from build123d import *

# Parameters (mm, degrees)
SKETCH_1_W               = 420
SKETCH_1_H               = 420
EXTRUDE_1_DEPTH          = 5
SKETCH_3_W               = 50
SKETCH_3_H               = 10
SKETCH_3_W_2             = 10
SKETCH_3_H_2             = 50
EXTRUDE_2_DEPTH          = 10
SKETCH_4_W               = 200
SKETCH_4_H               = 10
SKETCH_4_W_2             = 10
SKETCH_4_H_2             = 200
EXTRUDE_3_DEPTH          = 10
FILLET_1_R               = 5
SKETCH_5_R               = 2
CUT_EXTRUDE_1_DEPTH      = 422.366823564
SKETCH_6_R               = 2
CUT_EXTRUDE_2_DEPTH      = 375.733238451
CUT_EXTRUDE_3_DEPTH      = 422.366823564
CUT_EXTRUDE_3_DEPTH_BACK = 422.366823564
SKETCH_7_R               = 2
SKETCH_8_R               = 2
CUT_EXTRUDE_4_DEPTH      = 375.733238451
CUT_EXTRUDE_5_DEPTH      = 422.366823564
CUT_EXTRUDE_5_DEPTH_BACK = 422.366823564
SKETCH_9_R               = 2
SKETCH_10_R              = 2
CUT_EXTRUDE_6_DEPTH      = 375.733238451
CUT_EXTRUDE_7_DEPTH      = 422.366823564
CUT_EXTRUDE_7_DEPTH_BACK = 422.366823564
SKETCH_11_R              = 2
SKETCH_12_R              = 2
CUT_EXTRUDE_8_DEPTH      = 375.733238451
SCALE_1_SCALE            = 0.5


with BuildPart() as part:
    # 草图1 → 凸台-拉伸1 (new body)
    with BuildSketch(Plane.XY):
        Rectangle(SKETCH_1_W, SKETCH_1_H)
    extrude(amount=EXTRUDE_1_DEPTH)

    # 草图3 → 凸台-拉伸2 (add)
    with BuildSketch(Plane(origin=(0, 0, 0), x_dir=(-1, 0, 0), z_dir=(0, 0, -1))):
        with Locations((-130, -205)):
            Rectangle(SKETCH_3_W, SKETCH_3_H)
        with Locations((-205, -130)):
            Rectangle(SKETCH_3_W_2, SKETCH_3_H_2)
        with Locations((-205, 130)):
            Rectangle(SKETCH_3_W_2, SKETCH_3_H_2)
        with Locations((-130, 205)):
            Rectangle(SKETCH_3_W, SKETCH_3_H)
        with Locations((205, 130)):
            Rectangle(SKETCH_3_W_2, SKETCH_3_H_2)
        with Locations((130, 205)):
            Rectangle(SKETCH_3_W, SKETCH_3_H)
        with Locations((205, -130)):
            Rectangle(SKETCH_3_W_2, SKETCH_3_H_2)
        with Locations((130, -205)):
            Rectangle(SKETCH_3_W, SKETCH_3_H)
    extrude(amount=EXTRUDE_2_DEPTH)

    # 草图4 → 凸台-拉伸3 (add)
    with BuildSketch(Plane.XY.offset(5)):
        with Locations((0, -205)):
            Rectangle(SKETCH_4_W, SKETCH_4_H)
        with Locations((205, 0)):
            Rectangle(SKETCH_4_W_2, SKETCH_4_H_2)
        with Locations((0, 205)):
            Rectangle(SKETCH_4_W, SKETCH_4_H)
        with Locations((-205, 0)):
            Rectangle(SKETCH_4_W_2, SKETCH_4_H_2)
    extrude(amount=EXTRUDE_3_DEPTH)

    # 圆角1
    fillet_1_edges = [part.edges().sort_by_distance(p)[0] for p in [
        (-210, 0, 15),
        (-200, 0, 15),
        (0, -210, 15),
        (0, -200, 15),
        (0, 200, 15),
        (0, 210, 15),
        (200, 0, 15),
        (210, 0, 15),
        (200, -130, -10),
        (210, -130, -10),
        (130, 210, -10),
        (130, 200, -10),
        (200, 130, -10),
        (210, 130, -10),
        (-130, -210, -10),
        (-130, -200, -10),
        (-130, 210, -10),
        (-130, 200, -10),
        (-210, 130, -10),
        (-200, 130, -10),
        (-210, -130, -10),
        (-200, -130, -10),
        (130, -210, -10),
        (130, -200, -10),
    ]]
    fillet(fillet_1_edges, radius=FILLET_1_R - 0.0001)  # a hair under: the kernel refuses the full size

    # 草图5 → 切除-拉伸1 (cut, through all)
    with BuildSketch(Plane(origin=(0, 155, 0), x_dir=(1, 0, 0), z_dir=(0, 1, 0))):
        with Locations(Location((205, 5, 0), (0, 0, 270))):
            Circle(SKETCH_5_R)
    extrude(amount=-CUT_EXTRUDE_1_DEPTH, mode=Mode.SUBTRACT)

    # 草图6 → 切除-拉伸2 (cut, through all)
    with BuildSketch(Plane(origin=(0, 100, 0), x_dir=(1, 0, 0), z_dir=(0, 1, 0))):
        with Locations(Location((205, -10, 0), (0, 0, 270))):
            Circle(SKETCH_6_R)
    extrude(amount=-CUT_EXTRUDE_2_DEPTH, mode=Mode.SUBTRACT)

    # 草图7 → 切除-拉伸3 (cut, two sides: drawn at the far end of the back side and taken through both)
    with BuildSketch(Plane(origin=(155, 0, 0), x_dir=(0, 0, -1), z_dir=(1, 0, 0)).offset(-CUT_EXTRUDE_3_DEPTH_BACK)):
        with Locations((5, -205)):
            Circle(SKETCH_7_R)
    extrude(amount=CUT_EXTRUDE_3_DEPTH + CUT_EXTRUDE_3_DEPTH_BACK, mode=Mode.SUBTRACT)

    # 草图8 → 切除-拉伸4 (cut, through all)
    with BuildSketch(Plane(origin=(100, 0, 0), x_dir=(0, 0, -1), z_dir=(1, 0, 0))):
        with Locations((-10, -205)):
            Circle(SKETCH_8_R)
    extrude(amount=-CUT_EXTRUDE_4_DEPTH, mode=Mode.SUBTRACT)

    # 草图9 → 切除-拉伸5 (cut, two sides: drawn at the far end of the back side and taken through both)
    with BuildSketch(Plane.XZ.offset(155).offset(-CUT_EXTRUDE_5_DEPTH_BACK)):
        with Locations((-205, -5)):
            Circle(SKETCH_9_R)
    extrude(amount=CUT_EXTRUDE_5_DEPTH + CUT_EXTRUDE_5_DEPTH_BACK, mode=Mode.SUBTRACT)

    # 草图10 → 切除-拉伸6 (cut, through all)
    with BuildSketch(Plane.XZ.offset(100)):
        with Locations(Location((-205, 10, 0), (0, 0, 270))):
            Circle(SKETCH_10_R)
    extrude(amount=-CUT_EXTRUDE_6_DEPTH, mode=Mode.SUBTRACT)

    # 草图11 → 切除-拉伸7 (cut, two sides: drawn at the far end of the back side and taken through both)
    with BuildSketch(Plane.ZY.offset(155).offset(-CUT_EXTRUDE_7_DEPTH_BACK)):
        with Locations(Location((-5, 205, 0), (0, 0, 270))):
            Circle(SKETCH_11_R)
    extrude(amount=CUT_EXTRUDE_7_DEPTH + CUT_EXTRUDE_7_DEPTH_BACK, mode=Mode.SUBTRACT)

    # 草图12 → 切除-拉伸8 (cut, through all)
    with BuildSketch(Plane.ZY.offset(100)):
        with Locations((10, 205)):
            Circle(SKETCH_12_R)
    extrude(amount=-CUT_EXTRUDE_8_DEPTH, mode=Mode.SUBTRACT)


with BuildPart() as part_1:
    # 缩放比例1: scaled about (0, 0, 0)
    add(part.part.scale(SCALE_1_SCALE))


solid = part_1.part
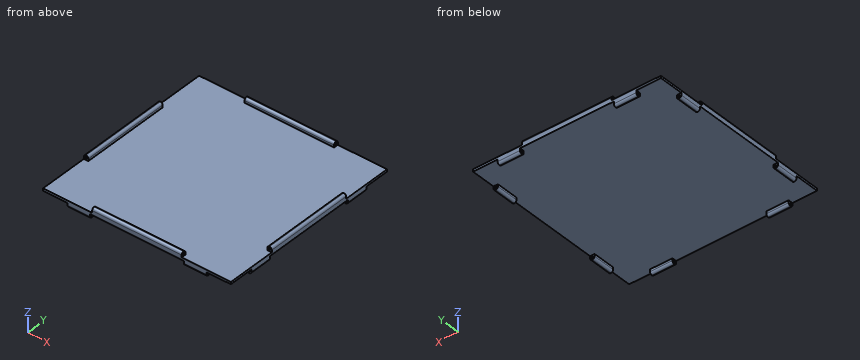
Geometry check sheet. Reference: the model listing, model coordinates, mm. Give positions to 0.01 mm unless a question says otherwise; leave off trailing zeros.
1. Scan lines: line 1 (X direction, y = 66.5, z = -2.5); line 2 (Y direction, x = 40, z = 3.5). Record each from-to range of solid material in increasing order.
Completed:
line 1: x = -105 to -103.5, -101.5 to -100, 100 to 101.5, 103.5 to 105
line 2: y = -105 to -100, 100 to 105
2. Depth check by flat-ended pin: pin 1 (1.5 mm diameter, centred on y = -101.5, z = -1.5, fed in from +X); pin 2 (2.5 mm diameter, centred on y = 102.5, z = 5, fed in from -X); pin 3 (2.5 mm diameter, centred on y = 102, z = -3, fed in from -X). Enter the tip coordinate at first touch or a pass-through.
Completed:
pin 1: stops at x = 77.5
pin 2: stops at x = -50
pin 3: stops at x = -77.5
3. Sectioned sample at A-A (x = 19.5). State how many separate pieces and enclosed holes the cut face has, then the cut area to 3 significant figures.
Completed:
separate pieces: 1
enclosed holes: 2
area: 563 mm2
